Autodesk Fusion 360 part; units mm, degrees
sketch "giraffe" plane through (0, 0, 0) normal (0, 0, 1) x (1, 0, 0)
  line L0 (-42.5977, 27.0275) -> (-55, 27.0275)
  line L1 (-55, 27.0275) -> (-55, 20)
  line L2 (-55, 20) -> (-65, 20)
  line L3 (-65, 20) -> (-65, 7.3444)
  line L4 (-65, 7.3444) -> (-55, 7.3444)
  line L5 (-55, 7.3444) -> (-55, 0)
  line L6 (-55, 0) -> (-35, 0)
  line L7 (-35, 0) -> (-35, -45)
  line L8 (-35, -45) -> (-22.9146, -45)
  line L9 (-22.9146, -45) -> (-22.9146, -37.0159)
  line L10 (-9.9884, -37.0159) -> (-9.9884, -45)
  line L11 (-9.9884, -45) -> (2.644, -45)
  line L12 (2.644, -45) -> (2.644, -25)
  line L13 (2.644, -25) -> (-3.6722, -25)
  line L14 (-3.6722, -25) -> (-3.6722, -17.0391)
  line L15 (-3.6722, -17.0391) -> (-9.9884, -17.0391)
  line L16 (-9.9884, -17.0391) -> (-9.9884, -25)
  line L17 (-22.9146, -25) -> (-22.9146, 40)
  line L18 (-22.9146, 40) -> (-30, 40)
  line L19 (-30, 40) -> (-30, 35)
  line L20 (-30, 35) -> (-35, 35)
  line L21 (-35, 35) -> (-35, 27.0275)
  line L22 (-35, 27.0275) -> (-42.5977, 27.0275)
  line L23 (-42.5977, 27.0275) -> (-42.5977, 40)
  line L24 (-42.5977, 40) -> (-35, 40)
  line L25 (-35, 40) -> (-35, 35)
  line L26 (-22.9146, 26.7337) -> (-15, 26.7337)
  line L27 (-15, 26.7337) -> (-15, 20)
  line L28 (-15, 20) -> (-10, 20)
  line L29 (-10, 20) -> (-10, 15)
  line L30 (-10, 15) -> (-15, 15)
  line L31 (-15, 15) -> (-15, 7.3444)
  line L32 (-15, 7.3444) -> (-10, 7.3444)
  line L33 (-10, 7.3444) -> (-10, 0)
  line L34 (-10, 0) -> (-15, 0)
  line L35 (-15, 0) -> (-15, -5)
  line L36 (-15, -5) -> (-10, -5)
  line L37 (-10, -5) -> (-10, -10)
  line L38 (-10, -10) -> (-15, -10)
  line L39 (-15, -10) -> (-15, -15)
  line L40 (-15, -15) -> (-15, -17.0391)
  line L41 (-15, -17.0391) -> (-9.9884, -17.0391)
  line L42 (-3.6722, -17.0391) -> (-3.6722, -12.5)
  line L43 (-3.6722, -12.5) -> (0, -12.5)
  line L44 (0, -12.5) -> (2.644, -12.5)
  line L45 (2.644, -12.5) -> (2.644, -25)
  line L46 (-35, -5) -> (-30, -5)
  line L47 (-30, -5) -> (-30, -12.5)
  line L48 (-30, -12.5) -> (-35, -12.5)
  line L49 (-30, -30) -> (-30, -37.0159)
  line L50 (-30, -37.0159) -> (-22.9146, -37.0159)
  line L51 (-22.9146, -37.0159) -> (-22.9146, -30)
  line L52 (-22.9146, -30) -> (-30, -30)
  line L53 (-9.9884, -37.0159) -> (-9.9884, -30)
  line L54 (-9.9884, -37.0159) -> (-3.6722, -37.0159)
  line L55 (-3.6722, -37.0159) -> (-3.6722, -30)
  line L56 (-3.6722, -30) -> (-9.9884, -30)
  line L57 (-42.5977, 7.5) -> (-35, 7.5)
  line L58 (-35, 7.5) -> (-35, 15)
  line L59 (-35, 15) -> (-42.5977, 15)
  line L60 (-42.5977, 15) -> (-42.5977, 7.5)
  line L61 (-42.5977, 15) -> (-42.5977, 20)
  line L62 (-42.5977, 20) -> (-50, 20)
  line L63 (-50, 20) -> (-50, 15)
  line L64 (-50, 15) -> (-42.5977, 15)
  line L65 (-35, -25) -> (-30, -25)
  line L66 (-30, -25) -> (-30, -17.0391)
  line L67 (-30, -17.0391) -> (-35, -17.0391)
  line L68 (-22.9146, -25) -> (-9.9884, -25)
  line L69 (-22.9146, -37.0159) -> (-9.9884, -37.0159)
extrude "Extrude1" add sketch "giraffe" along normal blind 10 contours L0 L1 L2 L3 L4 L5 L6 L7 L8 L9 L10 L11 L12 L13 L14 L15 L16 L17 L18 L19 L20 L21 L22 L46 L47 L48 L65 L66 L67 L68 L69 makes body 1
extrude "Extrude2" add sketch "giraffe" along normal blind 8 separate body contours L49 L50 L51 L52 | L53 L54 L55 L56 | L21 L22 L23 L24 L25 | L16 L17 L26 L27 L28 L29 L30 L31 L32 L33 L34 L35 L36 L37 L38 L39 L40 L41 L68 | L13 L14 L42 L43 L44 L45 makes body 2 at (-42.5977, 31.3517, 5.3333) makes body 3 at (-20.2764, 0.5779, 0) makes body 4 at (-27.6382, -37.0159, 2.6667) makes body 5 at (-3.6722, -20.8333, 5.3333) makes body 6 at (-9.9884, -34.6773, 2.6667)
combine "Combine1" operation add target body 5 tool bodies 2 3 1 6 4
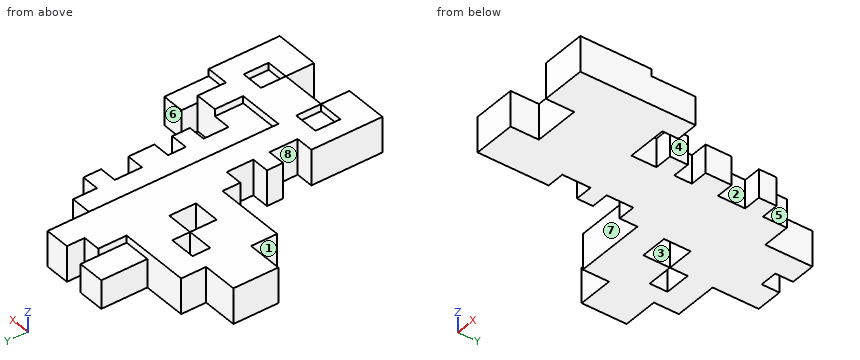
Model file for the job. Use its own axes, mm. Face numbers are marked on the shaded views. A direction names the side the tool comes from. Coordinates: 2 decimals unless noted, no trailing zeros. Write each loop counter-clockwise with the first axis right and the second up, starting at its lowest first coordinate (ties: lowest second). Pieces come first, ordered by that corner, then holes. Notation, with made-up numbers: (77.5, 70) - (83.5, 70) arc R22 ccw to (83.5, 97) - close; hole circle Ø8 at (24.25, 48.5). An arc over 180 degrees is marked (long way). Use a Markdown table: item, result. Add a question column.
Item 1: 3-axis set-ups, long thin cutter, end or side, ignore diameter. For the marked faces 1, 2, 3 and 4: which of +Z, -Z, +X, -X, +Y, -Y reach the whole face in a straight line?
Item 2: Drop flat-ended pins along their axis: pin 1 (2 mm diameter, centred on y = 4.5, z = 2, fed in from +X); pin 2 (1.9 mm diameter, centred on x = 0.5, y = -18, fed in from +Z); pin 3 (2.5 mm diameter, centred on y = -41.5, z = 6.5, fed in from -X); pin 4 (5.5 mm diameter, centred on x = -12.5, z = 4.5, fed in from -Y). Give the stop position or say it passes through.
Item 3: Band-saw the part on B-B, the plane y = -15. Write the cut outline in (x, z), and give its area (3 significant figures).
Item 4: Band-saw the part on A-A, the plane x = -47. Write the cut outline in (y, z).
Item 5: Two-plate mould, pull along Y, no slides. Class the marked faces 5, 6, 7 and 8: pulls with the +Y half, pulls with the -Y half, needs draft (parallel to the pull), parting line crosses it, or undercut.
Item 6: Drill centre lines: line 1 along Y through (x, z) = (-33, 7); line 2 along X through (y, z) = (-13, 4.5); line 3 along Y through (x, z) = (-44.5, 7.5). Where is each one in solid material? Low to high.
Item 7: Band-saw the part on D-D, the plane y = -4. Write the cut outline in (x, z), and give its area (3 significant figures).
Item 8: Band-saw the part on C-C, the plane x = -27.5. Write the cut outline in (y, z).
A:
| question | item | result |
|---|---|---|
| 1 | face 1 | +Z, -Z, -X, -Y |
| 1 | face 2 | +Z, -Z, +X |
| 1 | face 3 | +Z, -Z |
| 1 | face 4 | +Z, -Z, +X, +Y |
| 2 | pin 1 | stops at x = -10 |
| 2 | pin 2 | stops at z = 8 |
| 2 | pin 3 | stops at x = -35 |
| 2 | pin 4 | stops at y = -45 |
| 3 | outline | (-35, 0) - (-15, 0) - (-15, 8) - (-22.91, 8) - (-22.91, 10) - (-35, 10) - close; (-3.67, 0) - (2.64, 0) - (2.64, 8) - (-3.67, 8) - close |
| 3 | area | 235 mm² |
| 4 | outline | (0, 0) - (15, 0) - (15, 10) - (0, 10) - close; (20, 0) - (27.03, 0) - (27.03, 10) - (20, 10) - close |
| 5 | face 5 | needs draft |
| 5 | face 6 | pulls with the +Y half |
| 5 | face 7 | pulls with the -Y half |
| 5 | face 8 | undercut |
| 6 | line 1 | y = -45 to -25, -17.04 to -12.5, -5 to 35 |
| 6 | line 2 | x = -35 to -15, -3.67 to 2.64 |
| 6 | line 3 | y = 0 to 15, 20 to 27.03 |
| 7 | outline | (-35, 0) - (-15, 0) - (-15, 8) - (-22.91, 8) - (-22.91, 10) - (-35, 10) - close |
| 7 | area | 184 mm² |
| 8 | outline | (-45, 0) - (40, 0) - (40, 10) - (-30, 10) - (-30, 8) - (-37.02, 8) - (-37.02, 10) - (-45, 10) - close |
